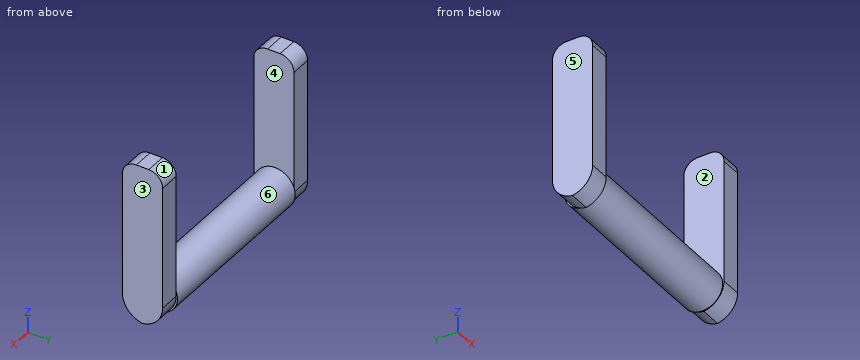
```python
from build123d import *

# Parameters (mm, degrees)
F0_R          = 1.8415
F1_DEPTH      = 16.51
F2_W          = 1.905
F2_H          = 3.683
F3_DEPTH      = 12.7
F3_DEPTH_BACK = 1.96215
F4_T1_DEPTH   = 12.7
F4_T3_DEPTH   = 7.3025
F4_T5_DEPTH   = 12.7
F4_T7_DEPTH   = 7.3025
F5_R          = 1.27


# Not quite as in the source:
# - a fillet or chamfer that OpenCascade refuses, or shapes differently, is made with other operations: its cross-section is extruded or revolved along the edge and cut away or added


with BuildPart() as f1:
    # F0 (on Right) → F1 (new body)
    with BuildSketch(Plane.YZ):
        Circle(F0_R)
    extrude(amount=F1_DEPTH)

    # F2 (on Top) → F3 (join, two sides)
    with BuildSketch(Plane.XY) as f3_sk:
        with Locations((17.4625, -0.1134487624)):
            Rectangle(F2_W, F2_H)
        with Locations((-0.9525, -0.1134487624)):
            Rectangle(F2_W, F2_H)
    extrude(amount=F3_DEPTH)
    extrude(f3_sk.sketch, amount=-F3_DEPTH_BACK)

    # F4: fillet of radius 2.159 on 4 edges, made by hand

    # F4_s2 → F4_t1 (cut)
    with BuildSketch(Plane.YZ.offset(11.1125)):
        with BuildLine():
            ThreePointArc((0.2040512376, -1.96215), (-1.322592303, -1.3297935406), (-1.9549487624, 0.19685))
            Line((-1.9549487624, 0.19685), (-1.9549487624, -1.96215))
            Line((-1.9549487624, -1.96215), (0.2040512376, -1.96215))
        make_face()
    extrude(amount=F4_T1_DEPTH, mode=Mode.SUBTRACT)

    # F4_s4 → F4_t3 (cut)
    with BuildSketch(Plane.YZ.offset(16.51)):
        with BuildLine():
            ThreePointArc((1.7280512376, 0.19685), (1.0956947782, -1.3297935406), (-0.4309487624, -1.96215))
            Line((-0.4309487624, -1.96215), (1.7280512376, -1.96215))
            Line((1.7280512376, -1.96215), (1.7280512376, 0.19685))
        make_face()
    extrude(amount=F4_T3_DEPTH, mode=Mode.SUBTRACT)

    # F4_s6 → F4_t5 (cut)
    with BuildSketch(Plane.YZ.offset(-7.3025)):
        with BuildLine():
            ThreePointArc((-1.9549487624, 0.19685), (-1.322592303, -1.3297935406), (0.2040512376, -1.96215))
            Line((0.2040512376, -1.96215), (-1.9549487624, -1.96215))
            Line((-1.9549487624, -1.96215), (-1.9549487624, 0.19685))
        make_face()
    extrude(amount=F4_T5_DEPTH, mode=Mode.SUBTRACT)

    # F4_s8 → F4_t7 (cut)
    with BuildSketch(Plane.YZ.offset(-7.3025)):
        with BuildLine():
            ThreePointArc((1.7280512376, 0.19685), (1.0956947782, -1.3297935406), (-0.4309487624, -1.96215))
            Line((-0.4309487624, -1.96215), (1.7280512376, -1.96215))
            Line((1.7280512376, -1.96215), (1.7280512376, 0.19685))
        make_face()
    extrude(amount=F4_T7_DEPTH, mode=Mode.SUBTRACT)

    # F5
    f5_edges = [f1.edges().sort_by_distance(p)[0] for p in [
        (-0.9525, -1.954949, 12.7),
        (-0.9525, 1.728051, 12.7),
        (17.4625, 1.728051, 12.7),
        (17.4625, -1.954949, 12.7),
    ]]
    fillet(f5_edges, radius=F5_R)


solid = f1.part
```
For this review, take the finished solid that the model builds, in its own axes (mm). Face numbers are marked on the shaded views. A direction names the side the tool comes from. Round coordinates to 2 decimals unless told otherwise and drop trailing zeros. Loops run counter-clockwise (first coordinate to the right, second up) from the corner with the lowest first, then second, coordinate; pieces in that order, holes last.
(1) We need section A-A (z = 4.5). Give the boundary of the cut face in (x, y) (3 decimals).
Returned:
outline: (-1.905, -1.955) - (0, -1.955) - (0, 1.728) - (-1.905, 1.728) - close; (16.51, -1.955) - (18.415, -1.955) - (18.415, 1.728) - (16.51, 1.728) - close
(2) We need section B-B (y = 1.25). Give the boundary of the cut face in (x, z) (3 decimals), plus the area to 3 significant figures.
Returned:
outline: (-1.905, -1.158) - (0, -1.158) - (0, -1.352) - (16.51, -1.352) - (16.51, -1.158) - (18.415, -1.158) - (18.415, 12.423) - (16.51, 12.423) - (16.51, 1.352) - (0, 1.352) - (0, 12.423) - (-1.905, 12.423) - close
area: 96.4 mm2
(3) Mouldability with a two-part tool opening along X and no side actions: class the marked faces 1, 2, 3 and 4 as released by +X, released by -X, zero draft, split by the parting line, or undercut.
Returned:
face 1: zero draft
face 2: undercut
face 3: released by +X
face 4: undercut
(4) Wall thickness on line 1 along X through (y, z) = (-0.15, 10.25) (3 decimals); line 2 along Y through (x, z) = (1.75, 0); line 3 along Z through (x, y) = (8, -1.45): over which ranges is each line inside the solid? List them lowest first.
Returned:
line 1: x = -1.905 to 0, 16.51 to 18.415
line 2: y = -1.84 to 1.84
line 3: z = -1.14 to 1.14
(5) We need section C-C (x = 0.25). Give the boundary of the cut face in (y, z), plus the area to 3 significant figures.
Returned:
outline: circle Ø3.68 at (0, 0)
area: 10.7 mm2
(6) We need section D-D (y = -1.15). Give the boundary of the cut face in (x, z) (3 decimals).
Returned:
outline: (-1.905, -1.485) - (0, -1.485) - (0, -1.438) - (16.51, -1.438) - (16.51, -1.485) - (18.415, -1.485) - (18.415, 12.612) - (16.51, 12.612) - (16.51, 1.438) - (0, 1.438) - (0, 12.612) - (-1.905, 12.612) - close
(7) Tool access review of the marked faces 5 and 6: name each direction out of +Z, -Z, +X, -X, +Y, -Y from which nothing blocks a thin tool from reaching the whole face with its end or side.
Returned:
face 5: +Z, -Z, -X, +Y, -Y
face 6: none
(8) Clearance check with flat-ended pins moving along their axes: P1, Ø6, axis at x = 8.5, z = 3.5, coming from the +Y side; P2, Ø1.5, axis at x = -1, z = 4.5, coming from the +Y side; P3, Ø0.7, axis at y = 1.5, z = -1, coming from the +X side (3 decimals). State where each tip first meets the part, or that it passes through.
Returned:
P1: stops at y = 1.77
P2: stops at y = 1.73
P3: stops at x = 18.415
